from build123d import *

# Parameters (mm, degrees)
SKETCH1_R           = 2.5
BOSS_EXTRUDE1_DEPTH = 2.8


with BuildPart() as part:
    # Sketch1 → Boss-Extrude1 (new body)
    with BuildSketch(Plane(origin=(0, 0, 0), x_dir=(1, 0, 0), z_dir=(0, 1, 0))):
        with BuildLine():
            Line((-1.3, -17.4), (-1.3, -10))
            Line((-1.3, -10), (1.3, -10))
            Line((1.3, -10), (1.3, -17.4))
            Line((1.3, -17.4), (5.136248173, -17.4))
            ThreePointArc((5.136248173, -17.4), (7.049665335, -17.019397663), (8.671782079, -15.935533906))
            Line((8.671782079, -15.935533906), (11.384419177, -13.222896808))
            Line((11.384419177, -13.222896808), (6.151828996, -7.990306627))
            Line((6.151828996, -7.990306627), (7.990306627, -6.151828996))
            Line((7.990306627, -6.151828996), (13.222896808, -11.384419177))
            Line((13.222896808, -11.384419177), (15.935533906, -8.671782079))
            ThreePointArc((15.935533906, -8.671782079), (17.019397663, -7.049665335), (17.4, -5.136248173))
            Line((17.4, -5.136248173), (17.4, -1.3))
            Line((17.4, -1.3), (10, -1.3))
            Line((10, -1.3), (10, 1.3))
            Line((10, 1.3), (17.4, 1.3))
            Line((17.4, 1.3), (17.4, 5.136248173))
            ThreePointArc((17.4, 5.136248173), (17.019397663, 7.049665335), (15.935533906, 8.671782079))
            Line((15.935533906, 8.671782079), (13.222896808, 11.384419177))
            Line((13.222896808, 11.384419177), (7.990306627, 6.151828996))
            Line((7.990306627, 6.151828996), (6.151828996, 7.990306627))
            Line((6.151828996, 7.990306627), (11.384419177, 13.222896808))
            Line((11.384419177, 13.222896808), (8.671782079, 15.935533906))
            ThreePointArc((8.671782079, 15.935533906), (7.049665335, 17.019397663), (5.136248173, 17.4))
            Line((5.136248173, 17.4), (1.3, 17.4))
            Line((1.3, 17.4), (1.3, 10))
            Line((1.3, 10), (-1.3, 10))
            Line((-1.3, 10), (-1.3, 17.4))
            Line((-1.3, 17.4), (-5.136248173, 17.4))
            ThreePointArc((-5.136248173, 17.4), (-7.049665335, 17.019397663), (-8.671782079, 15.935533906))
            Line((-8.671782079, 15.935533906), (-11.384419177, 13.222896808))
            Line((-11.384419177, 13.222896808), (-6.151828996, 7.990306627))
            Line((-6.151828996, 7.990306627), (-7.990306627, 6.151828996))
            Line((-7.990306627, 6.151828996), (-13.222896808, 11.384419177))
            Line((-13.222896808, 11.384419177), (-15.935533906, 8.671782079))
            ThreePointArc((-15.935533906, 8.671782079), (-17.019397663, 7.049665335), (-17.4, 5.136248173))
            Line((-17.4, 5.136248173), (-17.4, 1.3))
            Line((-17.4, 1.3), (-10, 1.3))
            Line((-10, 1.3), (-10, -1.3))
            Line((-10, -1.3), (-17.4, -1.3))
            Line((-17.4, -1.3), (-17.4, -5.136248173))
            ThreePointArc((-17.4, -5.136248173), (-17.019397663, -7.049665335), (-15.935533906, -8.671782079))
            Line((-15.935533906, -8.671782079), (-13.222896808, -11.384419177))
            Line((-13.222896808, -11.384419177), (-7.990306627, -6.151828996))
            Line((-7.990306627, -6.151828996), (-6.151828996, -7.990306627))
            Line((-6.151828996, -7.990306627), (-11.384419177, -13.222896808))
            Line((-11.384419177, -13.222896808), (-8.671782079, -15.935533906))
            ThreePointArc((-8.671782079, -15.935533906), (-7.049665335, -17.019397663), (-5.136248173, -17.4))
            Line((-5.136248173, -17.4), (-1.3, -17.4))
        make_face()
        with Locations(Location((0, 0, 0), (0, 0, 270))):  # turned: the seam where the file's is
            Circle(SKETCH1_R, mode=Mode.SUBTRACT)
    extrude(amount=BOSS_EXTRUDE1_DEPTH)


solid = part.part
Source: CAD feature listing. Evaluate the final solid. Frame: model axes, mm. A direction names the side the tool comes from. Round coordinates to 2 decimals unless told otherwise and drop trailing zeros. Loops run counter-clockwise (first coordinate to the right, second up) from the corner with the lowest first, then second, coordinate; pieces in that order, holes last.
Q1. Section B-B, the plane x = 0. Return loops of the section in (y, z).
Q2. Access query for faces 1 (the face through (-8.8, 1.38, -10.64)), 2 (the face through (14, 1, 1.3)), 3 (the face through (-14, 1, 1.3)). Directions: +Z, -Z, +X, -X, +Y, -Y. A direction counts if a zero-diameter tool reaches every point of the face in a straight line with its end or side. Return the directions, or none.
Q3. Section A-A, the plane z = 0. Return loops of the section in (x, y), plus the area to 3 significant figures.
Q4. Ray query, line 1 (Z direction, x = 9, y = 0.55); line 2 (X direction, y = 0.2, z = -8.5); line 3 (X direction, y = 1.4, z = 7). Return the intervals inside material, ascending.
Q5. Mould query, pull axis X, two halves, no side actions, for faces 4 (the face through (10.05, 1.38, -14.56)), 5 (the face through (-3, 1, -17.4)), 6 (the face through (1.3, 1, 14)). Classes: pulls with the +X half, pulls with the -X half, needs draft (parallel to the pull), parting line crosses it, or undercut.
Q6. First-contact query: P1, Ø0.8, axis at y = 2, z = 13.5, coming from the -X side; P2, Ø4, axis at x = 0, z = 0, coming from the -Y side; P3, Ø1.5, axis at y = 2, z = 10.5, coming from the +X side; P4, Ø1.3, axis at x = -0.5, y = 1.5, coming from the +Z side. Flat tips, straight axial feed; report the tip coordinate or a pass-through.
Solutions:
1. outline: (0, -10) - (2.8, -10) - (2.8, -2.5) - (0, -2.5) - close; (0, 2.5) - (2.8, 2.5) - (2.8, 10) - (0, 10) - close
2. face 1: +Y, -Y
2. face 2: +X, +Y, -Y
2. face 3: -X, +Y, -Y
3. outline: (-10, 0) - (-2.5, 0) - (-2.5, 2.8) - (-10, 2.8) - close; (2.5, 0) - (10, 0) - (10, 2.8) - (2.5, 2.8) - close
3. area: 42.0 mm2
4. line 1: z = -15.61 to -10.84, -7.16 to 7.16, 10.84 to 15.61
4. line 2: x = -16.1 to -10.34, -6.66 to 6.66, 10.34 to 16.1
4. line 3: x = -17.04 to -8.84, -7.14 to 7.14, 8.84 to 17.04
5. face 4: pulls with the +X half
5. face 5: needs draft
5. face 6: undercut
6. P1: stops at x = -11.38
6. P2: passes through
6. P3: stops at x = 14.86
6. P4: stops at z = 10
